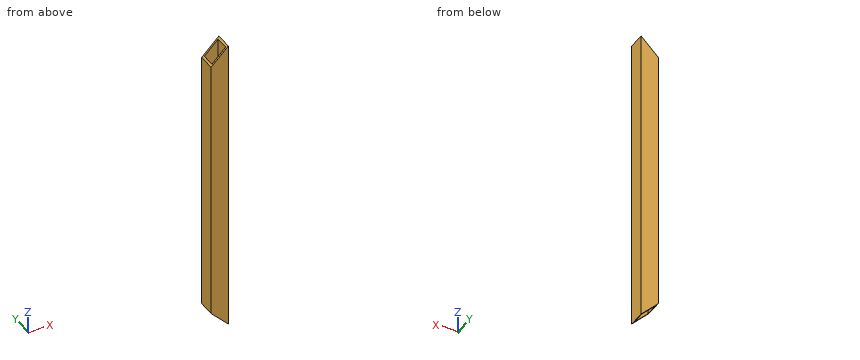
from build123d import *

# Parameters (mm, degrees)
SKETCH1_W          = 40
SKETCH1_H          = 40
SKETCH1_W_2        = 32
SKETCH1_H_2        = 32
CUT_EXTRUDE1_DEPTH = 41.0000001


with BuildPart() as part:
    # Sweep1: sweep along a curve in space
    with BuildLine() as sweep1_path:
        add(Edge.make_bspline(
            [(0, 0, 0), (0, 0, 700)],
            knots=[0, 0, 1, 1], degree=1))
    # Sketch1 → Sweep1 (sweep)
    with BuildSketch(Plane.XY):
        Rectangle(SKETCH1_W, SKETCH1_H)
        Rectangle(SKETCH1_W_2, SKETCH1_H_2, mode=Mode.SUBTRACT)
    sweep(path=sweep1_path.line)

    # Sketch2 → Cut-Extrude1 (cut, through all)
    with BuildSketch(Plane(origin=(0, 20, 0), x_dir=(1, 0, 0), z_dir=(0, 1, 0))):
        Polygon((20, 0), (-20, -40), (-20, 0), align=None)
        Polygon((20, -700), (-20, -660), (-20, -700), align=None)
    extrude(amount=-CUT_EXTRUDE1_DEPTH, mode=Mode.SUBTRACT)


solid = part.part
Work out the finished part from the listing and answer in its coordinate system (mm). Give positions to 0.01 mm unless a question says otherwise; leave off trailing zeros. Order: outer loops, then holes, each group sorted by start corner. A loop starts at its lowest first (then second) coordinate and runs counter-clockwise, first axis right, second up. Notation, with made-up numbers: (35, -34) -> (79, -34) arc R35 cw to (79, 1) -> close; hole circle Ø4 at (16, 10). An arc over 180 degrees is marked (long way). Answer as a JSON object with one key per item and string values. Group by question number.
1. A flat-ended cylindrical pin translates along its axis: pin 1 Ø6 at (x, y) = (4, 15.5) entering from +Z. Find the tip coordinate at first contact, or state that the pin passes through.
2. Section C-C on z = 444.5 is taken. Determine the outline of the cut face in (x, y), plus the area to 3 significant figures.
3. Consider line 1 along Y through (x, z) = (2.5, 246); line 2 along X through (y, z) = (-4, 672.5). Determine where each line is inside the solid, lowest interval first. Write a range as [from, to].
4. Section B-B on y = -8.5 is taken. Determine the outline of the cut face in (x, z).
5. Section A-A on x = 8 is taken. Determine the outline of the cut face in (y, z), plus the area to 3 significant figures.
Result sheet:
{
 "1": {"pin 1": "stops at z = 686.96"},
 "2": {"outline": "(-20, -20) -> (20, -20) -> (20, 20) -> (-20, 20) -> close; hole (-16, -16) -> (16, -16) -> (16, 16) -> (-16, 16) -> close", "area": "576 mm^2"},
 "3": {"line 1": "y = [-20, -16], [16, 20]", "line 2": "x = [16, 20]"},
 "4": {"outline": "(-20, 40) -> (-16, 36) -> (-16, 664) -> (-20, 660) -> close; (16, 4) -> (20, 0) -> (20, 700) -> (16, 696) -> close"},
 "5": {"outline": "(-20, 12) -> (-16, 12) -> (-16, 688) -> (-20, 688) -> close; (16, 12) -> (20, 12) -> (20, 688) -> (16, 688) -> close", "area": "5,410 mm^2"}
}
